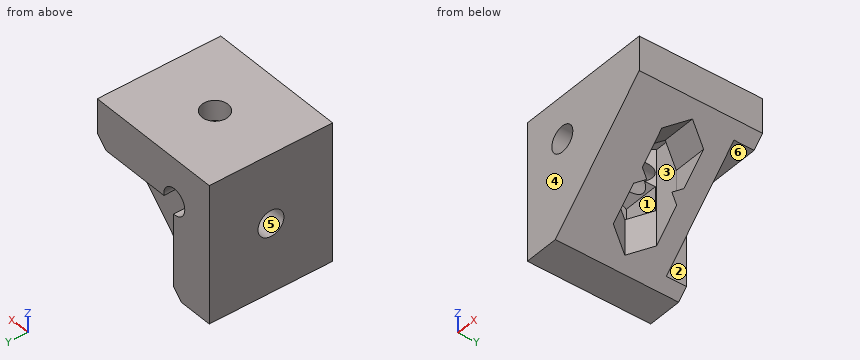
```python
from build123d import *

# Parameters (mm, degrees)
MAIN_BODY_DEPTH              = 34
SKETCH3_R                    = 3.571875
F_9_32_RIGHT_RAIL_DEPTH      = 1
F_9_32_RIGHT_RAIL_DEPTH_BACK = 5.55625
SKETCH4_R                    = 3.571875
F_9_32_LEFT_RAIL_DEPTH       = 5.55625
SKETCH8_R                    = 3.571875
F_9_32_TOPPER_DEPTH          = 1
F_9_32_TOPPER_DEPTH_BACK     = 35
CUT_EXTRUDE3_START           = -5.55625
CUT_EXTRUDE3_DEPTH           = 32.54375
CUT_EXTRUDE4_START           = -5.55625
CUT_EXTRUDE4_DEPTH           = 32.54375
CUT_EXTRUDE6_DEPTH           = 5.55625


with BuildPart() as part:
    # Sketch1 → Main Body (new body)
    with BuildSketch(Plane(origin=(0, 0, 0), x_dir=(1, 0, 0), z_dir=(0, 1, 0))):
        Polygon((0, 0), (38.1, 0), (38.1, 9.525), (9.525, 38.1), (0, 38.1), align=None)
    extrude(amount=MAIN_BODY_DEPTH)

    # Sketch3 → 9/32 Right Rail (cut, two sides)
    with BuildSketch(Plane.XY) as f_9_32_right_rail_sk:
        with Locations((19.05, 17)):
            Circle(SKETCH3_R)
    extrude(amount=F_9_32_RIGHT_RAIL_DEPTH, mode=Mode.SUBTRACT)
    extrude(f_9_32_right_rail_sk.sketch, amount=-F_9_32_RIGHT_RAIL_DEPTH_BACK, mode=Mode.SUBTRACT)

    # Sketch4 → 9/32 Left Rail (cut)
    with BuildSketch(Plane.ZY):
        with Locations((-19.05, 17)):
            Circle(SKETCH4_R)
    extrude(amount=-F_9_32_LEFT_RAIL_DEPTH, mode=Mode.SUBTRACT)

    # Sketch8 → 9/32 Topper (cut, two sides)
    with BuildSketch(Plane(origin=(0, 34, 0), x_dir=(1, 0, 0), z_dir=(0, 1, 0))) as f_9_32_topper_sk:
        with Locations((11.90625, 11.90625)):
            Circle(SKETCH8_R)
    extrude(amount=F_9_32_TOPPER_DEPTH, mode=Mode.SUBTRACT)
    extrude(f_9_32_topper_sk.sketch, amount=-F_9_32_TOPPER_DEPTH_BACK, mode=Mode.SUBTRACT)

    # Sketch9 → Cut-Extrude3 (cut)
    with BuildSketch(Plane.ZY.offset(CUT_EXTRUDE3_START)):
        Polygon((-22.372470377, 22.7546875), (-25.694940754, 17), (-22.372470377, 11.2453125), (-15.727529623, 11.2453125), (-12.405059246, 17), (-15.727529623, 22.7546875), align=None)
    extrude(amount=-CUT_EXTRUDE3_DEPTH, mode=Mode.SUBTRACT)

    # Sketch10 → Cut-Extrude4 (cut)
    with BuildSketch(Plane.XY.offset(CUT_EXTRUDE4_START)):
        Polygon((15.612961679, 22.953125), (12.175923357, 17), (15.612961679, 11.046875), (22.487038321, 11.046875), (25.924076643, 17), (22.487038321, 22.953125), align=None)
    extrude(amount=-CUT_EXTRUDE4_DEPTH, mode=Mode.SUBTRACT)

    # Sketch13 → Cut-Extrude6 (cut)
    with BuildSketch(Plane(origin=(0, 34, 0), x_dir=(1, 0, 0), z_dir=(0, 1, 0))):
        Polygon((35.219940754, 12.405059246), (12.175923357, 12.405059246), (12.175923357, 35.449076643), align=None)
    extrude(amount=-CUT_EXTRUDE6_DEPTH, mode=Mode.SUBTRACT)


solid = part.part
```
Could you check a few things on this model? Use its own coordinates, in mm. Face numbers are marked on the shaded views. A direction names the side the tool comes from. Round coordinates to 2 decimals unless told otherwise and drop trailing zeros. Write each loop counter-clockwise with the first axis right and the second up, starting at its lowest first coordinate (ties: lowest second). Pieces come first, ordered by that corner, then holes. Notation, with made-up numbers: M 42.5,62 L 59.5,62 A15 cw 59.5,79 Z; hole C 17,2.25 d7. An arc over 180 degrees is marked long. Answer in a Markdown table with one row per item. Add a question column.
Q1. Will these pins go through, and if not, where does the flat tip stop? pin 1 Ø8 at (y, z) = (10, -25) entering from -X; pin 2 Ø6 at (x, y) = (24.5, 24.5) entering from -Z (3 decimals); pin 3 Ø1.5 at (x, y) = (29.5, 19) entering from -Z; pin 4 Ø7.5 at (x, z) = (26, -19) entering from +Y.
Q2. On a 3-axis mill with a long thin cutter (end or side, diameter ignored), from which of +Z, -Z, +X, -X, +Y, -Y can I reach the whole of each face in a straight line? I mean the marked faces 1, 2 and 3. Say none if no direction works.
Q3. Imagine slicing it at B-B (y = 12.5). Please give me the cut outline in (x, z) (3 decimals).
Q4. If I drill on line 1 (Y direction, x = 12.5, z = -21.5); line 2 (Y direction, x = 4, z = -19); line 3 (Z direction, x = 20.5, y = 12), over which ranges is the centre line in solid material (lowest first)? Write a range as from..to.
Q5. Imagine slicing it at C-C (x = 19.05). Please give me the cut outline in (y, z) (3 decimals).
Q6. If we mould it in two halves opening along Y, with no side actions, what happens to the marked faces 4, 5 and 6? For each: +Y half, -Y half, draft (parallel to the pull), parting line (faces both ways), or undercut.
Q7. Imagine slicing it at D-D (z = -19.05). Please give me the cut outline in (x, y) (3 decimals).
Q8. Imagine slicing it at A-A (z = -7). Please give me the cut outline in (x, y), then the cut area to 3 significant figures.
Values:
| question | item | result |
|---|---|---|
| 1 | pin 1 | x = 0 |
| 1 | pin 2 | z = -26.125 |
| 1 | pin 3 | z = -13.99 |
| 1 | pin 4 | y = 28.44 |
| 2 | face 1 | +X |
| 2 | face 2 | -Z, +X, +Y |
| 2 | face 3 | -Z |
| 3 | outline | M 0,-38.1 L 9.525,-38.1 L 14.774,-32.851 L 14.774,-23.097 L 5.556,-23.097 L 5.556,-15.003 L 10.126,-15.003 A3.572 cw long 14.774,-9.777 L 14.774,-5.556 L 23.326,-5.556 L 23.326,-15.003 L 32.622,-15.003 L 38.1,-9.525 L 38.1,0 L 0,0 Z; M 13.686,-15.003 L 14.774,-15.003 L 14.774,-14.036 A3.572 cw Z; M 23.326,-24.299 L 24.528,-23.097 L 23.326,-23.097 Z |
| 4 | line 1 | 0..11.25, 22.75..28.44 |
| 4 | line 2 | 0..13.43, 20.57..34 |
| 4 | line 3 | -5.56..0 |
| 5 | outline | M 0,-28.575 L 11.047,-28.575 L 11.047,-5.556 L 13.428,-5.556 L 13.428,0 L 0,0 Z; M 20.572,-5.556 L 22.953,-5.556 L 22.953,-28.575 L 28.444,-28.575 L 28.444,-12.405 L 34,-12.405 L 34,0 L 20.572,0 Z |
| 6 | face 4 | -Y half |
| 6 | face 5 | undercut |
| 6 | face 6 | draft |
| 7 | outline | M 0,0 L 28.575,0 L 28.575,11.245 L 22.602,11.245 L 22.487,11.047 L 15.613,11.047 L 15.498,11.245 L 5.556,11.245 L 5.556,13.428 L 0,13.428 Z; M 0,20.572 L 5.556,20.572 L 5.556,22.755 L 15.498,22.755 L 15.613,22.953 L 22.487,22.953 L 22.602,22.755 L 28.575,22.755 L 28.575,28.444 L 12.176,28.444 L 12.176,34 L 0,34 Z |
| 8 | outline | M 0,0 L 38.1,0 L 38.1,34 L 0,34 Z; hole M 12.18,17 L 15.61,11.05 L 22.49,11.05 L 25.92,17 L 22.49,22.95 L 15.61,22.95 Z |
| 8 | area | 1,170 mm^2 |
